Input: part model. Units: mm. Frame: model coordinates. Coordinates: 2 decimals unless noted, no trailing zeros. Write each loop counter-clockwise with the first axis right and the second up, starting at its lowest first coordinate (ties: lowest second). Pieces come first, ordered by that corner, then holes. Notation, with made-up numbers: M 70,34 L 116,34 A7 ccw 116,39 Z; hole C -36,55.25 d6. An arc over 180 degrees is marked long. Answer as a JSON object with one key per item and string values. Group by question number.
Autodesk Inventor part; units mm, degrees
ref_plane "YZ Plane" through (0, 0, 0) normal (1, 0, 0) x (0, 1, 0)
ref_plane "XZ Plane" through (0, 0, 0) normal (0, 1, 0) x (-1, 0, 0)
ref_plane "XY Plane" through (0, 0, 0) normal (0, 0, 1) x (1, 0, 0)
sketch "Sketch1" plane through (0, 0, 0) normal (0, 1, 0) x (-1, 0, 0)
  circle A0 centre (0, 0) radius 1.5
  line L0 (0.74, -1.3048) -> (7.523, 2.5423)
  line L1 (5.523, 3.1933) -> (-0.4244, 1.4387)
  line L2 (5.523, 3.1933) -> (7.523, 4.5423)
  line L3 (7.523, 4.5423) -> (7.523, 2.5423)
  line L4 (7.523, 3.5) -> (7.523, 4.5)
  line L5 (7.4579, 4.5004) -> (6.1505, 3.6591)
  point P0 (7.523, 3.5423)
  dimension "d2" = 3
  dimension "d4" = 2
  dimension "d7" = 7.523
  dimension "d8" = 4.5423
  dimension "d9" = 56
  dimension "d10" = 2
extrude "Extrusion1" add sketch "Sketch1" along normal mid plane 2
sketch "Sketch2" plane through (0, -1, 0) normal (0, 1, 0) x (1, 0, 0)
  arc A0 (0.4244, -1.4387) -> (-0.74, 1.3048) centre (0, 0) ccw
  circle A1 centre (0, 0) radius 1.5
extrude "Extrusion2" add sketch "Sketch2" against normal blind 5
properties part number "Pawl"
Q1. Pin query (flat end, axial travel): pin 1 Ø4 at (x, y) = (-4, -1.5) entering from +Z; pin 2 Ø2 at (x, y) = (-2, -2.5) entering from -Z; pin 3 Ø1.8 at (x, z) = (-3, 2.5) entering from -Y. Return the tip coordinate at first contact, or that it passes through.
Q2. Line query: line 1 (Y direction, x = -2, z = -0.5); line 2 (X direction, y = -2.5, z = 0); line 3 (X direction, y = 0.25, z = 4.25). Output: solid intervals per line, ascending. Write a range as from..to.
Q3. Section A-A, the plane y = -0.5. Return the cut outline in (x, z), and give its area (3 significant figures).
Q4. Section D-D, the plane x = -5.75. Return the cut outline in (y, z).
Q5. Section B-B, the plane z = 0. Return the cut outline in (x, y), and give its area (3 significant figures).
Filled in:
{
 "1": {"pin 1": "z = 3.47", "pin 2": "z = -1.12", "pin 3": "y = -1"},
 "2": {"line 1": "-1..1", "line 2": "-1.5..1.5", "line 3": "-7.52..-7.09"},
 "3": {"outline": "M -7.52,2.54 L -0.74,-1.3 A1.5 ccw long 0.42,1.44 L -5.52,3.19 L -7.52,4.54 Z", "area": "21.3 mm^2"},
 "4": {"outline": "M -1,1.54 L 1,1.54 L 1,3.35 L -1,3.35 Z"},
 "5": {"outline": "M -3.04,-1 L -1.5,-1 L -1.5,-6 L 1.5,-6 L 1.5,1 L -3.04,1 Z", "area": "24.1 mm^2"}
}
